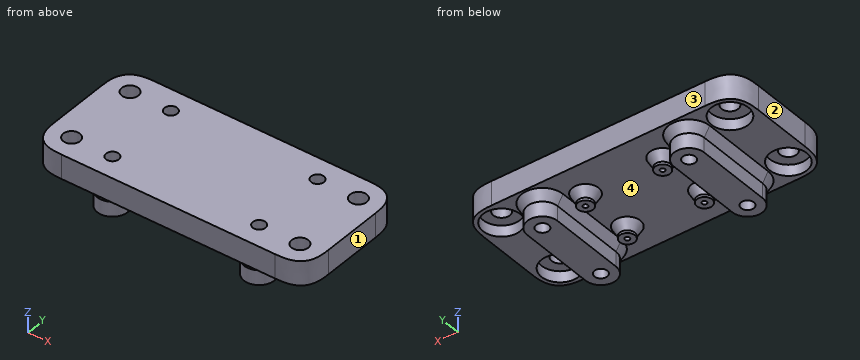
from build123d import *

# Parameters (mm, degrees)
SKETCH1_R                                    = 2.5
BOSS_EXTRUDE1_DEPTH                          = 4
BOSS_EXTRUDE1_2_DEPTH                        = 4
BOSS_EXTRUDE1_3_DEPTH                        = 4
BOSS_EXTRUDE1_4_DEPTH                        = 4
SKETCH2_W                                    = 90.48
SKETCH2_H                                    = 40
BOSS_EXTRUDE2_DEPTH                          = 8
CBORE_FOR_M5_HEX_HEAD_CAP_SCREW1_D           = 5.5
CBORE_FOR_M5_HEX_HEAD_CAP_SCREW1_CBORE_D     = 12.24
CBORE_FOR_M5_HEX_HEAD_CAP_SCREW1_CBORE_DEPTH = 3.65
F_1_16_0_0625_DIAMETER_HOLE1_D               = 1.5875
F_1_16_0_0625_DIAMETER_HOLE1_DEPTH           = 7
F_1_16_0_0625_DIAMETER_HOLE1_TIP             = 0.476933116
FILLET1_SIZE                                 = 10
BOSS_EXTRUDE3_DEPTH                          = 8
M5X0_8_TAPPED_HOLE2_D                        = 4.2
CHAMFER1_SIZE                                = 1.8
CHAMFER1_SIZE2                               = 3.117691454


with BuildPart() as part:
    # Sketch1 → Boss-Extrude1 (new body)
    with BuildSketch(Plane.XY):
        with Locations((12.75, 8.94)):
            Circle(SKETCH1_R)
    extrude(amount=BOSS_EXTRUDE1_DEPTH)



with BuildPart() as body_2:
    # Sketch1 → Boss-Extrude1 2 (new body)
    with BuildSketch(Plane.XY):
        with Locations((12.75, -8.94)):
            Circle(SKETCH1_R)
    extrude(amount=BOSS_EXTRUDE1_2_DEPTH)


with BuildPart() as body_3:
    # Sketch1 → Boss-Extrude1 3 (new body)
    with BuildSketch(Plane.XY):
        with Locations((-12.75, -8.94)):
            Circle(SKETCH1_R)
    extrude(amount=BOSS_EXTRUDE1_3_DEPTH)


with BuildPart() as body_4:
    # Sketch1 → Boss-Extrude1 4 (new body)
    with BuildSketch(Plane.XY):
        with Locations((-12.75, 8.94)):
            Circle(SKETCH1_R)
    extrude(amount=BOSS_EXTRUDE1_4_DEPTH)


with BuildPart() as part_1:
    add(part.part)

    add(body_2.part)  # Boss-Extrude2 merges body 2

    add(body_3.part)  # Boss-Extrude2 merges body 3

    add(body_4.part)  # Boss-Extrude2 merges body 4
    # Sketch2 → Boss-Extrude2 (add)
    with BuildSketch(Plane.XY.offset(4)):
        Rectangle(SKETCH2_W, SKETCH2_H)
    extrude(amount=BOSS_EXTRUDE2_DEPTH)

    # CBORE for M5 Hex Head Cap Screw1 (through all)
    with Locations(Plane(origin=(0, 0, 4), x_dir=(-1, 0, 0), z_dir=(0, 0, -1))):
        with Locations((37.74, 12.5), (-37.74, -12.5), (-37.74, 12.5), (37.74, -12.5)):
            CounterBoreHole(CBORE_FOR_M5_HEX_HEAD_CAP_SCREW1_D / 2, CBORE_FOR_M5_HEX_HEAD_CAP_SCREW1_CBORE_D / 2, CBORE_FOR_M5_HEX_HEAD_CAP_SCREW1_CBORE_DEPTH)

    # 1/16 (0.0625) Diameter Hole1
    with Locations(Plane(origin=(0, 0, 0), x_dir=(-1, 0, 0), z_dir=(0, 0, -1))):
        with Locations((-12.75, -8.94), (-12.75, 8.94), (12.75, -8.94), (12.75, 8.94)):
            Hole(F_1_16_0_0625_DIAMETER_HOLE1_D / 2, depth=F_1_16_0_0625_DIAMETER_HOLE1_DEPTH)
            with Locations((0, 0, -(F_1_16_0_0625_DIAMETER_HOLE1_DEPTH + F_1_16_0_0625_DIAMETER_HOLE1_TIP / 2))):  # 118° drill point
                Cone(0, F_1_16_0_0625_DIAMETER_HOLE1_D / 2, F_1_16_0_0625_DIAMETER_HOLE1_TIP, mode=Mode.SUBTRACT)

    # Fillet1
    # a fillet whose section is not a circle: 10 mm, written as the material it takes off along each edge
    with BuildSketch(Plane(origin=(-45.24, -20, -21), x_dir=(0, 1, 0), z_dir=(0, 0, 1)), Plane(origin=(-45.24, 20, -21), x_dir=(1, 0, 0), z_dir=(0, 0, 1))) as fillet1_piece_1:
        with BuildLine():
            add(Edge.make_bspline([(FILLET1_SIZE, 0), (FILLET1_SIZE * 0.831801948466, 0), (FILLET1_SIZE * 0.663603896932, 0), (FILLET1_SIZE * 0.292893218813, -FILLET1_SIZE * 0.0716919198361), (FILLET1_SIZE * 0.0716919198361, -FILLET1_SIZE * 0.292893218813), (0, -FILLET1_SIZE * 0.663603896932), (0, -FILLET1_SIZE * 0.831801948466), (0, -FILLET1_SIZE)], knots=[0, 0, 0, 0, 0, 0, 0.5, 0.5, 1, 1, 1, 1, 1, 1], degree=5))
            Line((0, -FILLET1_SIZE), (0, 0))
            Line((0, 0), (FILLET1_SIZE, 0))
        make_face()
    extrude(amount=58, mode=Mode.SUBTRACT)
    with BuildSketch(Plane(origin=(45.24, 20, -21), x_dir=(-1, 0, 0), z_dir=(0, 0, 1)), Plane(origin=(45.24, -20, -21), x_dir=(0, 1, 0), z_dir=(0, 0, 1))) as fillet1_piece_2:
        with BuildLine():
            add(Edge.make_bspline([(FILLET1_SIZE, 0), (FILLET1_SIZE * 0.831801948466, 0), (FILLET1_SIZE * 0.663603896932, 0), (FILLET1_SIZE * 0.292893218813, FILLET1_SIZE * 0.0716919198361), (FILLET1_SIZE * 0.0716919198361, FILLET1_SIZE * 0.292893218813), (0, FILLET1_SIZE * 0.663603896932), (0, FILLET1_SIZE * 0.831801948466), (0, FILLET1_SIZE)], knots=[0, 0, 0, 0, 0, 0, 0.5, 0.5, 1, 1, 1, 1, 1, 1], degree=5))
            Line((0, FILLET1_SIZE), (0, 0))
            Line((0, 0), (FILLET1_SIZE, 0))
        make_face()
    extrude(amount=58, mode=Mode.SUBTRACT)

    # Sketch13 → Boss-Extrude3 (add)
    with BuildSketch(Plane(origin=(0, 0, 4), x_dir=(-1, 0, 0), z_dir=(0, 0, -1))):
        with BuildLine():
            Line((-19.24, 12.5), (-19.24, -12.5))
            ThreePointArc((-19.24, -12.5), (-24.24, -17.5), (-29.24, -12.5))
            Line((-29.24, -12.5), (-29.24, 12.5))
            ThreePointArc((-29.24, 12.5), (-24.24, 17.5), (-19.24, 12.5))
        make_face()
    boss_extrude3 = extrude(amount=BOSS_EXTRUDE3_DEPTH)

    # M5x0.8 Tapped Hole2 (through all)
    with Locations(Plane(origin=(0, 0, -4), x_dir=(-1, 0, 0), z_dir=(0, 0, -1))):
        with Locations((-24.24, -12.5), (-24.24, 12.5)):
            m5x0_8_tapped_hole2 = Hole(M5X0_8_TAPPED_HOLE2_D / 2)

    # Mirror2: Boss-Extrude3, M5x0.8 Tapped Hole2 across plane
    add(boss_extrude3.mirror(Plane(origin=(0, 0, 0), x_dir=(0, 0, 1), z_dir=(1, 0, 0))))
    add(m5x0_8_tapped_hole2.mirror(Plane(origin=(0, 0, 0), x_dir=(0, 0, 1), z_dir=(1, 0, 0))), mode=Mode.SUBTRACT)

    # Chamfer1
    chamfer1_edges = [part_1.edges().sort_by_distance(p)[0] for p in [
        (24.24, 17.5, 4),
        (29.24, 0, 4),
        (24.24, -17.5, 4),
        (19.24, 0, 4),
        (-24.24, 17.5, 4),
        (-29.24, 0, 4),
        (-24.24, -17.5, 4),
        (-19.24, 0, 4),
        (10.25, -8.94, 4),
        (-15.25, -8.94, 4),
        (-15.25, 8.94, 4),
        (10.25, 8.94, 4),
    ]]
    chamfer1_side = [part_1.faces().sort_by_distance(p)[0] for p in [
        (0, -1.03e-07, 4),
    ]]
    chamfer(chamfer1_edges, length=CHAMFER1_SIZE, length2=CHAMFER1_SIZE2, reference=chamfer1_side[0])


solid = part_1.part
The model under review builds one solid part; all positions refer to its coordinate system, in mm. Face numbers are marked on the shaded views. Give positions to 0.01 mm unless a question says otherwise; leave off trailing zeros. Loops run counter-clockwise (first coordinate to the right, second up) from the corner with the lowest first, then second, coordinate; pieces in that order, holes last. Notation, with made-up numbers: (78, 11.5) -> (107, 11.5) arc R14 ccw to (107, 33.5) -> close; hole circle Ø10 at (57.5, 52.5). An arc over 180 degrees is marked (long way). Answer as a JSON object with one key per item and string values. Group by question number.
Q1. Draft analysis for pull direction X (two halves, no side actions). For the marked faces 1, 2, 3 and 4, state which applies: pulls with the +X half, pulls with the -X half, needs draft (parallel to the pull), parting line crosses it, or undercut.
Q2. Insertion check: pin 1 (4 mm diameter, centred on y = -1, z = -2, fed in from -X); pin 2 (1.4 mm diameter, centred on x = -12.75, y = -8.94, fed in from -Z); pin 3 (2 mm diameter, centred on x = -34.5, y = 2, fed in from -Z); pin 4 (3.5 mm diameter, centred on x = -24.24, y = 12.5, fed in from +Z). Each pin has a flat end and moves straight along its axis. Give the tip position at first contact, or say it passes through.
Q3. Wall thickness on line 1 along Y through (x, z) = (12.75, 4.5); line 2 along Y through (x, z) = (24.24, -0.5); line 3 along X through (y, z) = (13, 7): over which ranges is each line inside the solid? List them lowest first.
Q4. Take a section at B-B (z = 10.75). State how many separate pieces and enclosed holes the cut face has, plus the area to 3 significant figures.
Q5. Take a section at A-A (x = -24.24). Write out the cut boundary in (y, z).
Q6. Take a section at C-C (x = -1). Write out the cut boundary in (y, z).
Answer below:
{
 "1": {"face 1": "pulls with the +X half", "face 2": "pulls with the -X half", "face 3": "needs draft", "face 4": "undercut"},
 "2": {"pin 1": "stops at x = -29.24", "pin 2": "stops at z = 7.06", "pin 3": "stops at z = 4", "pin 4": "passes through"},
 "3": {"line 1": "y = -20 to -9.73, -8.15 to 8.15, 9.73 to 20", "line 2": "y = -17.5 to -14.6, -10.4 to 10.4, 14.6 to 17.5", "line 3": "x = -45.11 to -43.84, -31.64 to -26.28, -22.2 to 22.2, 26.28 to 31.64, 43.84 to 45.11"},
 "4": {"separate pieces": "1", "enclosed holes": "8", "area": "3,420 mm2"},
 "5": {"outline": "(-20, 4) -> (-19.3, 4) -> (-17.5, 0.88) -> (-17.5, -4) -> (-14.6, -4) -> (-14.6, 12) -> (-20, 12) -> close; (-10.4, -4) -> (10.4, -4) -> (10.4, 12) -> (-10.4, 12) -> close; (14.6, -4) -> (17.5, -4) -> (17.5, 0.88) -> (19.3, 4) -> (20, 4) -> (20, 12) -> (14.6, 12) -> close"},
 "6": {"outline": "(-20, 4) -> (20, 4) -> (20, 12) -> (-20, 12) -> close"}
}
